```python
from build123d import *

# Parameters (mm, degrees)
EXTRUDE_1_DEPTH      = 14
CUT_EXTRUDE_1_DEPTH  = 44
SKETCH_8_W           = 5
SKETCH_8_H           = 44
CUT_EXTRUDE_2_DEPTH  = 10
SKETCH_9_W           = 25
SKETCH_9_H           = 44
EXTRUDE_2_DEPTH      = 10
SKETCH_10_W          = 50
SKETCH_10_H          = 7
CUT_EXTRUDE_3_DEPTH  = 10
SKETCH_11_W          = 6.2
SKETCH_11_H          = 7
CUT_EXTRUDE_4_DEPTH  = 10
SKETCH_12_W          = 5
SKETCH_12_H          = 5
SKETCH_12_W_2        = 20
SKETCH_12_H_2        = 20
EXTRUDE_3_DEPTH      = 45
SKETCH_13_W          = 5
SKETCH_13_H          = 7.5
EXTRUDE_4_DEPTH      = 10
SKETCH_14_W          = 15
SKETCH_14_H          = 10
EXTRUDE_5_DEPTH      = 5
SKETCH_15_R          = 1.55
CUT_EXTRUDE_5_DEPTH  = 5
CUT_EXTRUDE_6_DEPTH  = 5
CUT_EXTRUDE_7_DEPTH  = 5
EXTRUDE_6_DEPTH      = 5
EXTRUDE_START        = -5
EXTRUDE_7_DEPTH      = 5
SKETCH_20_W          = 0.2
SKETCH_20_H          = 20
CUT_EXTRUDE_8_DEPTH  = 45
CUT_EXTRUDE_START    = -100
CUT_EXTRUDE_9_DEPTH  = 100
CUT_EXTRUDE_10_DEPTH = 100
SKETCH_24_R          = 1.55
CUT_EXTRUDE_11_DEPTH = 100
SKETCH_25_R          = 3
SKETCH_25_R_2        = 1.55
CUT_EXTRUDE_12_DEPTH = 2
CUT_EXTRUDE_START_2  = -2
SKETCH_26_R          = 3
CUT_EXTRUDE_13_DEPTH = 2
CUT_EXTRUDE_14_DEPTH = 5
SKETCH_28_R          = 3
CUT_EXTRUDE_15_DEPTH = 2


with BuildPart() as part:
    # 草图1 → 凸台-拉伸1 (new body)
    with BuildSketch(Plane.XY):
        Polygon((-15, 22), (-15, -22), (15, -22), (15, 22), (0, 22), align=None)
    extrude(amount=EXTRUDE_1_DEPTH)

    # 草图2 → 切除-拉伸1 (cut)
    with BuildSketch(Plane(origin=(0, 22, 0), x_dir=(1, 0, 0), z_dir=(0, 1, 0))):
        Polygon((-15, 0), (-15, -14), (-10, -4), (-3.1, -4), (-3.1, 0), align=None)
        Polygon((3.1, -4), (10, -4), (15, -14), (15, 0), (3.1, 0), align=None)
    extrude(amount=-CUT_EXTRUDE_1_DEPTH, mode=Mode.SUBTRACT)

    # 草图8 → 切除-拉伸2 (cut)
    with BuildSketch(Plane(origin=(0, 0, 4), x_dir=(-1, 0, 0), z_dir=(0, 0, -1))):
        with Locations((-12.5, 0)):
            Rectangle(SKETCH_8_W, SKETCH_8_H)
    extrude(amount=-CUT_EXTRUDE_2_DEPTH, mode=Mode.SUBTRACT)

    # 草图9 → 凸台-拉伸2 (add)
    with BuildSketch(Plane(origin=(0, 0, 4), x_dir=(-1, 0, 0), z_dir=(0, 0, -1))):
        with Locations((-22.5, 0)):
            Rectangle(SKETCH_9_W, SKETCH_9_H)
    extrude(amount=-EXTRUDE_2_DEPTH)

    # 草图10 → 切除-拉伸3 (cut)
    with BuildSketch(Plane(origin=(0, 0, 4), x_dir=(-1, 0, 0), z_dir=(0, 0, -1))):
        with Locations((-10, -18.5)):
            Rectangle(SKETCH_10_W, SKETCH_10_H)
        with Locations((-10, 18.5)):
            Rectangle(SKETCH_10_W, SKETCH_10_H)
    extrude(amount=-CUT_EXTRUDE_3_DEPTH, mode=Mode.SUBTRACT)

    # 草图11 → 切除-拉伸4 (cut)
    with BuildSketch(Plane(origin=(0, 0, 0), x_dir=(-1, 0, 0), z_dir=(0, 0, -1))):
        with Locations((0, 18.5)):
            Rectangle(SKETCH_11_W, SKETCH_11_H)
        with Locations((0, -18.5)):
            Rectangle(SKETCH_11_W, SKETCH_11_H)
    extrude(amount=-CUT_EXTRUDE_4_DEPTH, mode=Mode.SUBTRACT)

    # 草图12 → 凸台-拉伸3 (add)
    with BuildSketch(Plane(origin=(0, 0, 4), x_dir=(-1, 0, 0), z_dir=(0, 0, -1))):
        with Locations((-32.5, 12.5)):
            Rectangle(SKETCH_12_W, SKETCH_12_H)
        with Locations((-20, 12.5)):
            Rectangle(SKETCH_12_W_2, SKETCH_12_H)
        with Locations((-32.5, 0)):
            Rectangle(SKETCH_12_W, SKETCH_12_H_2)
        with Locations((-32.5, -12.5)):
            Rectangle(SKETCH_12_W, SKETCH_12_H)
        with Locations((-20, -12.5)):
            Rectangle(SKETCH_12_W_2, SKETCH_12_H)
    extrude(amount=EXTRUDE_3_DEPTH)

    # 草图13 → 凸台-拉伸4 (add)
    with BuildSketch(Plane(origin=(0, 15, 0), x_dir=(1, 0, 0), z_dir=(0, 1, 0))):
        with Locations((12.5, 27.25)):
            Rectangle(SKETCH_13_W, SKETCH_13_H)
        with Locations((12.5, 19.75)):
            Rectangle(SKETCH_13_W, SKETCH_13_H)
    extrude(amount=EXTRUDE_4_DEPTH)

    # 草图14 → 凸台-拉伸5 (add)
    with BuildSketch(Plane.ZY.offset(-10)):
        with Locations((-23.5, -20)):
            Rectangle(SKETCH_14_W, SKETCH_14_H)
    extrude(amount=-EXTRUDE_5_DEPTH)

    # 草图15 → 切除-拉伸5 (cut)
    with BuildSketch(Plane.ZY.offset(-10)):
        with Locations((-23.5, 20)):
            Circle(SKETCH_15_R)
        with Locations((-23.5, -20)):
            Circle(SKETCH_15_R)
    extrude(amount=-CUT_EXTRUDE_5_DEPTH, mode=Mode.SUBTRACT)

    # 草图16 → 切除-拉伸6 (cut)
    with BuildSketch(Plane.ZY.offset(-10)):
        with BuildLine():
            Line((-31, 25), (-31, 20))
            ThreePointArc((-31, 20), (-29.535533906, 23.535533906), (-26, 25))
            Line((-26, 25), (-31, 25))
        make_face()
        with BuildLine():
            Line((-16, 25), (-21, 25))
            ThreePointArc((-21, 25), (-17.464466094, 23.535533906), (-16, 20))
            Line((-16, 20), (-16, 25))
        make_face()
    extrude(amount=-CUT_EXTRUDE_6_DEPTH, mode=Mode.SUBTRACT)

    # 草图17 → 切除-拉伸7 (cut)
    with BuildSketch(Plane.ZY.offset(-10)):
        with BuildLine():
            ThreePointArc((-26, -25), (-29.535533906, -23.535533906), (-31, -20))
            Line((-31, -20), (-31, -25))
            Line((-31, -25), (-26, -25))
        make_face()
        with BuildLine():
            ThreePointArc((-16, -20), (-17.464466094, -23.535533906), (-21, -25))
            Line((-21, -25), (-16, -25))
            Line((-16, -25), (-16, -20))
        make_face()
    extrude(amount=-CUT_EXTRUDE_7_DEPTH, mode=Mode.SUBTRACT)

    # 草图18 → 凸台-拉伸6 (add)
    with BuildSketch(Plane.XZ.offset(15)):
        with BuildLine():
            Line((10, -41), (10, -31))
            ThreePointArc((10, -31), (7.071067812, -38.071067812), (0, -41))
            Line((0, -41), (10, -41))
        make_face()
    extrude(amount=-EXTRUDE_6_DEPTH)

    # 草图19 → 凸台-拉伸7 (add)
    with BuildSketch(Plane(origin=(0, 15, 0), x_dir=(1, 0, 0), z_dir=(0, 1, 0)).offset(EXTRUDE_START)):
        with BuildLine():
            Line((10, 41), (0, 41))
            ThreePointArc((0, 41), (7.071067812, 38.071067812), (10, 31))
            Line((10, 31), (10, 41))
        make_face()
    extrude(amount=EXTRUDE_7_DEPTH)

    # 草图20 → 切除-拉伸8 (cut)
    with BuildSketch(Plane(origin=(0, 0, -41), x_dir=(-1, 0, 0), z_dir=(0, 0, -1))):
        with Locations((-30.1, 0)):
            Rectangle(SKETCH_20_W, SKETCH_20_H)
    extrude(amount=-CUT_EXTRUDE_8_DEPTH, mode=Mode.SUBTRACT)

    # 草图21 → 切除-拉伸9 (cut)
    with BuildSketch(Plane(origin=(0, 15, 0), x_dir=(1, 0, 0), z_dir=(0, 1, 0)).offset(CUT_EXTRUDE_START)):
        with BuildLine():
            Line((10, 41), (0, 41))
            ThreePointArc((0, 41), (7.071067812, 38.071067812), (10, 31))
            Line((10, 31), (10, 41))
        make_face()
    extrude(amount=CUT_EXTRUDE_9_DEPTH, mode=Mode.SUBTRACT)

    # 草图23 → 切除-拉伸10 (cut)
    with BuildSketch(Plane.XZ.offset(-10)):
        with BuildLine():
            ThreePointArc((21.65, -18.5), (21.401225478, -17.657793223), (20.73475838, -17.085934302))
            Line((20.73475838, -17.085934302), (19.46524162, -19.914065698))
            ThreePointArc((19.46524162, -19.914065698), (20.942206777, -19.801225478), (21.65, -18.5))
        make_face()
        with BuildLine():
            Line((19.46524162, -19.914065698), (20.73475838, -17.085934302))
            ThreePointArc((20.73475838, -17.085934302), (18.685934302, -17.86524162), (19.46524162, -19.914065698))
        make_face()
    extrude(amount=-CUT_EXTRUDE_10_DEPTH, mode=Mode.SUBTRACT)

    # 草图24 → 切除-拉伸11 (cut)
    with BuildSketch(Plane(origin=(0, 15, 0), x_dir=(1, 0, 0), z_dir=(0, 1, 0)).offset(CUT_EXTRUDE_START)):
        with Locations(Location((20.1, 18.5, 0), (0, 0, 90))):
            Circle(SKETCH_24_R)
    extrude(amount=CUT_EXTRUDE_11_DEPTH, mode=Mode.SUBTRACT)

    # 草图25 → 切除-拉伸12 (cut)
    with BuildSketch(Plane.XZ.offset(15)):
        with Locations(Location((20.1, -18.5, 0), (0, 0, 270))):
            Circle(SKETCH_25_R)
        with Locations(Location((20.1, -18.5, 0), (0, 0, 90))):
            Circle(SKETCH_25_R_2, mode=Mode.SUBTRACT)
    extrude(amount=-CUT_EXTRUDE_12_DEPTH, mode=Mode.SUBTRACT)

    # 草图26 → 切除-拉伸13 (cut)
    with BuildSketch(Plane(origin=(0, 15, 0), x_dir=(1, 0, 0), z_dir=(0, 1, 0)).offset(CUT_EXTRUDE_START_2)):
        with Locations(Location((20.1, 18.5, 0), (0, 0, 90))):
            Circle(SKETCH_26_R)
    extrude(amount=CUT_EXTRUDE_13_DEPTH, mode=Mode.SUBTRACT)

    # 草图27 → 切除-拉伸14 (cut)
    with BuildSketch(Plane(origin=(35, 0, 0), x_dir=(0, 0, -1), z_dir=(1, 0, 0))):
        with BuildLine():
            ThreePointArc((25.05, 0), (24.596015511, 1.096015511), (23.5, 1.55))
            Line((23.5, 1.55), (23.5, 0))
            Line((23.5, 0), (25.05, 0))
        make_face()
        with BuildLine():
            Line((25.05, 0), (23.5, 0))
            Line((23.5, 0), (23.5, -1.55))
            ThreePointArc((23.5, -1.55), (24.596015511, -1.096015511), (25.05, 0))
        make_face()
        with BuildLine():
            Line((23.5, 0), (23.5, 1.55))
            ThreePointArc((23.5, 1.55), (21.95, 0), (23.5, -1.55))
            Line((23.5, -1.55), (23.5, 0))
        make_face()
    extrude(amount=-CUT_EXTRUDE_14_DEPTH, mode=Mode.SUBTRACT)

    # 草图28 → 切除-拉伸15 (cut)
    with BuildSketch(Plane(origin=(35, 0, 0), x_dir=(0, 0, -1), z_dir=(1, 0, 0))):
        with Locations(Location((23.5, 0, 0), (0, 0, 90))):
            Circle(SKETCH_28_R)
    extrude(amount=-CUT_EXTRUDE_15_DEPTH, mode=Mode.SUBTRACT)


solid = part.part
```
Check sheet for the modelled part. Datum: model origin and axes. Units: mm. A direction names the side the tool comes from. Round coordinates to 2 decimals unless told otherwise and drop trailing zeros. Loops run counter-clockwise (first coordinate to the right, second up) from the corner with the lowest first, then second, coordinate; pieces in that order, holes last. Notation, with made-up numbers: (13, -24.75) -> (49, -24.75) arc R26 ccw to (49, -1.75) -> close; hole circle Ø2 at (12.25, 51). An arc over 180 degrees is marked (long way). Answer in a Markdown table with one row per item.
Q1. Sectioned sample at C-C on z = -3. Enter the section's corners in (x, y), then the cut area to 3 significant figures.
Data:
| item | result |
|---|---|
| outline | (10, -15) -> (35, -15) -> (35, 15) -> (10, 15) -> (10, 10) -> (30.2, 10) -> (30.2, -10) -> (10, -10) -> close |
| area | 346 mm^2 |
Q2. Sectioned sample at A-A on y = 14. Enter the section's corners in (x, z).
Data:
| item | result |
|---|---|
| outline | (-15, 14) -> (-10, 4) -> (-3.1, 4) -> (-3.1, 0) -> (3.1, 0) -> (3.1, 4) -> (10, 4) -> (10, -41) -> (35, -41) -> (35, 14) -> close; hole circle Ø6 at (20.1, -18.5) |
Q3. Sectioned sample at B-B on y = -4.5. Enter the section's corners in (x, z).
Data:
| item | result |
|---|---|
| outline | (-15, 14) -> (-10, 4) -> (-3.1, 4) -> (-3.1, 0) -> (3.1, 0) -> (3.1, 4) -> (30.2, 4) -> (30.2, -41) -> (35, -41) -> (35, 14) -> close |
Q4. Thickness scan on L1, parallel to Y at x = 11.9, z = -23.5; L2, parallel to Y at x = 27.5, z = -6; L3, parallel to Z at x = 33.85, y = 0. Record the ranges inside material, lowest first.
Data:
| item | result |
|---|---|
| L1 | y = -25 to -21.55, -18.45 to -10, 10 to 18.45, 21.55 to 25 |
| L2 | y = -15 to -10, 10 to 15 |
| L3 | z = -41 to -26.5, -20.5 to 14 |
Q5. Set-up check for faces 1 (the face through (12, 17, -16)), 2 (the face through (15, 19.9, -21.7)), 3 (the face through (19, -13, -20)), 4 (the face through (12, -18, -31)): record each of +Z, -Z, +X, -X, +Y, -Y from which the full face is reachable in a straight line by a thin tool's end or side.
Data:
| item | result |
|---|---|
| face 1 | +Z, +X, -X, +Y |
| face 2 | +Z, -Z, +X, +Y |
| face 3 | -Y |
| face 4 | -Z, +X, -X, -Y |
Q6. Go/stop test with flat-tipped pins: P1, Ø1.9, axis at y = -20, z = -23.5, coming from the -X side; P2, Ø5.5, axis at x = 20.1, z = -18.5, coming from the +Y side; P3, Ø5.5, axis at x = -6, y = 1.5, coming from the -Z side; P4, Ø2.5, axis at x = 12, y = 17, coming from the -Z side. Record where each tip stops, or that it passes through.
Data:
| item | result |
|---|---|
| P1 | passes through |
| P2 | stops at y = 13 |
| P3 | stops at z = 4 |
| P4 | stops at z = -31 |
Q7. Release check for a two-part mould opening along X. For faces 5 (the face through (15, -19.9, -25.3)), 6 (the face through (-12.535, 0.21, 9.07)), 7 (the face through (21, 13, -20)) record: released by +X, released by -X, zero draft, split by the parting line, or undercut.
Data:
| item | result |
|---|---|
| face 5 | released by +X |
| face 6 | released by -X |
| face 7 | undercut |
Q8. Sectioned sample at D-D on x = 4. Enter the section's corners in (y, z).
Data:
| item | result |
|---|---|
| outline | (-15, 4) -> (15, 4) -> (15, 14) -> (-15, 14) -> close |
